Could you check a few things on this model? Use its own coordinates, in mm. Face numbers are marked on the shaded views. Round coordinates to 2 decimals unless told otherwise and drop trailing zeros. Loops run counter-clockwise (first coordinate to the right, second up) from the corner with the lowest first, then second, coordinate; pieces in that order, holes last. Notation, with made-up numbers: (29.25, 8) -> (38.25, 8) arc R12 cw to (38.25, 21) -> close; hole circle Ø6 at (20, 26). An arc over 180 degrees is marked (long way). One line per item, written item: value.
```python
from build123d import *

# Parameters (mm, degrees)
BOSS_EXTRUDE1_START = 0.1
SKETCH1_W           = 3.71
SKETCH1_H           = 5.8
BOSS_EXTRUDE1_DEPTH = 2.55
SKETCH2_W           = 0.45
SKETCH2_H           = 1.82
BOSS_EXTRUDE2_DEPTH = 0.5
SKETCH3_W           = 0.88
SKETCH3_H           = 4
CUT_EXTRUDE1_DEPTH  = 0.7


with BuildPart() as part:
    # Sketch1 → Boss-Extrude1 (new body)
    with BuildSketch(Plane(origin=(0, 0, 0), x_dir=(1, 0, 0), z_dir=(0, 1, 0)).offset(BOSS_EXTRUDE1_START)):
        Rectangle(SKETCH1_W, SKETCH1_H)
    extrude(amount=BOSS_EXTRUDE1_DEPTH)

    # Sketch2 → Boss-Extrude2 (add)
    with BuildSketch(Plane(origin=(0, 0, 0), x_dir=(1, 0, 0), z_dir=(0, 1, 0))):
        with Locations((0.635, -3.31)):
            Rectangle(SKETCH2_W, SKETCH2_H)
        with Locations((-0.635, -3.31)):
            Rectangle(SKETCH2_W, SKETCH2_H)
        with Locations((-0.635, 3.31)):
            Rectangle(SKETCH2_W, SKETCH2_H)
        with Locations((0.635, 3.31)):
            Rectangle(SKETCH2_W, SKETCH2_H)
    extrude(amount=BOSS_EXTRUDE2_DEPTH)

    # Sketch3 → Cut-Extrude1 (cut)
    with BuildSketch(Plane(origin=(0, 2.65, 0), x_dir=(1, 0, 0), z_dir=(0, 1, 0))):
        with Locations((-0.635, 0)):
            Rectangle(SKETCH3_W, SKETCH3_H)
        with Locations((0.635, 0)):
            Rectangle(SKETCH3_W, SKETCH3_H)
    extrude(amount=-CUT_EXTRUDE1_DEPTH, mode=Mode.SUBTRACT)


solid = part.part
```
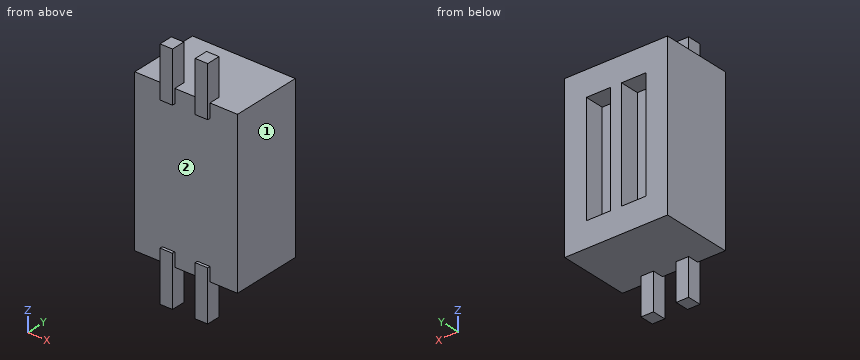
Item 1: Will these pins go through, and if not, where does the flat tip stop? pin 1 Ø0.8 at (x, y) = (0, 2) entering from -Z; pin 2 Ø0.5 at (x, z) = (-0.5, -4) entering from +Y; pin 3 Ø1.5 at (x, y) = (0.5, 2.5) entering from +Z.
Output:
pin 1: stops at z = -2.9
pin 2: stops at y = 0.5
pin 3: stops at z = 2.9
Item 2: If we section it at A-A on z = -3: List the corners of the cut face in (x, y) for me, plus the area to 3 significant figures.
Output:
outline: (-0.86, 0) -> (-0.41, 0) -> (-0.41, 0.5) -> (-0.86, 0.5) -> close; (0.41, 0) -> (0.86, 0) -> (0.86, 0.5) -> (0.41, 0.5) -> close
area: 0.450 mm²
Item 3: I need wall thicknesses on line 1 (X direction, y = 2.35, z = -0.75) (3 decimals); line 2 (Z direction, x = 0.4, y = 2.2); line 3 (Y direction, x = 1.4, z = 0.25). Which ranges of each line are inside material? Lowest first, please. Write a range as from..to.
Output:
line 1: x = -1.855..-1.075, -0.195..0.195, 1.075..1.855
line 2: z = -2.9..-2, 2..2.9
line 3: y = 0.1..2.65
Item 4: If we section it at C-C on x = -0.6: List the corners of the cut face in (y, z) for me.
Output:
outline: (0, -4.22) -> (0.5, -4.22) -> (0.5, -2.9) -> (2.65, -2.9) -> (2.65, -2) -> (1.95, -2) -> (1.95, 2) -> (2.65, 2) -> (2.65, 2.9) -> (0.5, 2.9) -> (0.5, 4.22) -> (0, 4.22) -> (0, 2.4) -> (0.1, 2.4) -> (0.1, -2.4) -> (0, -2.4) -> close
Item 5: If we mould it in two halves opening along Z, with no side actions, what happens to the marked faces 1 and 2? For each: released by +Z, released by -Z, zero draft, split by the parting line, or undercut.
Output:
face 1: zero draft
face 2: undercut
Item 6: If we section it at D-D on z = 2.5: List the corners of the cut face in (x, y) for me (3 decimals), plus the area to 3 significant figures.
Output:
outline: (-1.855, 0.1) -> (-0.86, 0.1) -> (-0.86, 0) -> (-0.41, 0) -> (-0.41, 0.1) -> (0.41, 0.1) -> (0.41, 0) -> (0.86, 0) -> (0.86, 0.1) -> (1.855, 0.1) -> (1.855, 2.65) -> (-1.855, 2.65) -> close
area: 9.55 mm²
Item 7: If we section it at B-B on y = 2.05: List the corners of the cut face in (x, z) for me (3 decimals), plus the area to 3 significant figures.
Output:
outline: (-1.855, -2.9) -> (1.855, -2.9) -> (1.855, 2.9) -> (-1.855, 2.9) -> close; hole (-1.075, -2) -> (-0.195, -2) -> (-0.195, 2) -> (-1.075, 2) -> close; hole (0.195, -2) -> (1.075, -2) -> (1.075, 2) -> (0.195, 2) -> close
area: 14.5 mm²
